from build123d import *

# Parameters (mm, degrees)
F0_R     = 2.5
F1_DEPTH = 25
F2_W     = 53.529413
F2_H     = 84.025737
F3_DEPTH = 22.8


with BuildPart() as f1:
    # F0 (on Top) → F1 (new body)
    with BuildSketch(Plane.XY):
        with Locations((22.5, 60.855222)):
            Circle(F0_R)
        with Locations((30, 53.355222)):
            Circle(F0_R)
        with Locations((30, 23.355222)):
            Circle(F0_R)
        with Locations((30, 8.355222)):
            Circle(F0_R)
        with Locations((22.5, 30.855222)):
            Circle(F0_R)
        with Locations((37.5, 60.855222)):
            Circle(F0_R)
        with Locations((22.5, 15.855222)):
            Circle(F0_R)
        with Locations((22.5, 0.855222)):
            Circle(F0_R)
        with Locations((37.5, 45.855222)):
            Circle(F0_R)
        with Locations((37.5, 15.855222)):
            Circle(F0_R)
        with Locations((22.5, 45.855222)):
            Circle(F0_R)
        with Locations((30, 38.355222)):
            Circle(F0_R)
        with Locations((37.5, 30.855222)):
            Circle(F0_R)
        with Locations((45, 53.355222)):
            Circle(F0_R)
        with Locations((45, 38.355222)):
            Circle(F0_R)
        with Locations((45, 23.355222)):
            Circle(F0_R)
        with Locations((37.5, 0.855222)):
            Circle(F0_R)
        with Locations((45, 8.355222)):
            Circle(F0_R)
        with Locations((52.5, 15.855222)):
            Circle(F0_R)
        with Locations((52.5, 30.855222)):
            Circle(F0_R)
        with Locations((52.5, 45.855222)):
            Circle(F0_R)
        with Locations((15, 53.355222)):
            Circle(F0_R)
        with Locations((15, 38.355222)):
            Circle(F0_R)
        with Locations((15, 23.355222)):
            Circle(F0_R)
        with Locations((15, 8.355222)):
            Circle(F0_R)
        with Locations((7.5, 15.855222)):
            Circle(F0_R)
        with Locations((7.5, 30.855222)):
            Circle(F0_R)
        with Locations((7.5, 45.855222)):
            Circle(F0_R)
    extrude(amount=F1_DEPTH)

    # F2 (on Top) → F3 (join)
    with BuildSketch(Plane.XY):
        with Locations((31.011025, 29.531249)):
            Rectangle(F2_W, F2_H)
    extrude(amount=-F3_DEPTH)


solid = f1.part
Verification items for the finished model (mm, model axes). A direction names the side the tool comes from. Coordinates: 2 decimals unless noted, no trailing zeros. Order: outer loops, then holes, each group sorted by start corner. A loop starts at its lowest first (then second) coordinate and runs counter-clockwise, first axis right, second up.
Item 1: Section check D-D, the plane x = 22.5. Enter the section's corners in (y, z).
Filled in:
outline: (-12.48, -22.8) - (71.54, -22.8) - (71.54, 0) - (63.36, 0) - (63.36, 25) - (58.36, 25) - (58.36, 0) - (48.36, 0) - (48.36, 25) - (43.36, 25) - (43.36, 0) - (33.36, 0) - (33.36, 25) - (28.36, 25) - (28.36, 0) - (18.36, 0) - (18.36, 25) - (13.36, 25) - (13.36, 0) - (3.36, 0) - (3.36, 25) - (-1.64, 25) - (-1.64, 0) - (-12.48, 0) - close
Item 2: Access from +Z, -Z, +X, -X, +Y, -Y to the whole of each face (thin tool, end or side, straight path). Record for faces 1 (the face through (12.502, 8.465, 12.325)), 2 (the face through (15, 38, 25)).
Filled in:
face 1: +Z
face 2: +Z, +X, -X, +Y, -Y
Item 3: Section check A-A, the plane z = 2.5. Give the number of separate pieces and of enclosed holes in the cut face, then the cut area to 3 significant figures.
Filled in:
separate pieces: 28
enclosed holes: 0
area: 550 mm2
Item 4: Material ranges on L1, parallel to X at y = 46, z = 13.5; L2, parallel to Y at x = 39.5, z = 14.5; L3, parallel to Y at x = 14, z = 4.5, recorded low to high.
Filled in:
L1: x = 5 to 10, 20 to 25, 35 to 40, 50 to 55
L2: y = -0.64 to 2.36, 14.36 to 17.36, 29.36 to 32.36, 44.36 to 47.36, 59.36 to 62.36
L3: y = 6.06 to 10.65, 21.06 to 25.65, 36.06 to 40.65, 51.06 to 55.65
Item 5: Release check for a two-part mould opening along Y. For faces 3 (the face through (31, 71.544, -11)), 4 (the face through (13.157, 55.045, 12.325)), 5 (the face through (45, 23, 25)) record: +Y half, -Y half, draft (parallel to the pull), parting line (faces both ways), or undercut.
Filled in:
face 3: +Y half
face 4: undercut
face 5: draft
Item 6: Section check C-C, the plane y = 66.5. Enter the section's corners in (x, z).
Filled in:
outline: (4.25, -22.8) - (57.78, -22.8) - (57.78, 0) - (4.25, 0) - close
Item 7: Depth check by flat-ended pin: pin 1 (12 mm diameter, centred on x = 46, y = 34, fed in from +Z); pin 2 (1.5 mm diameter, centred on x = 25, z = 7.5, fed in from +Y); pin 3 (1 mm diameter, centred on y = 39.5, z = 8, fed in from +X). Enter the tip coordinate at first touch or a pass-through.
Filled in:
pin 1: stops at z = 25
pin 2: stops at y = 62.64
pin 3: stops at x = 47.42
Item 8: Section check B-B, the plane x = 15. Enter the section's corners in (y, z), then the cut area to 3 significant figures.
Filled in:
outline: (-12.48, -22.8) - (71.54, -22.8) - (71.54, 0) - (55.86, 0) - (55.86, 25) - (50.86, 25) - (50.86, 0) - (40.86, 0) - (40.86, 25) - (35.86, 25) - (35.86, 0) - (25.86, 0) - (25.86, 25) - (20.86, 25) - (20.86, 0) - (10.86, 0) - (10.86, 25) - (5.86, 25) - (5.86, 0) - (-12.48, 0) - close
area: 2,420 mm2
